Input: part model. Units: mm. Frame: model coordinates. Face numbers are marked on the shaded views. A direction names the side the tool comes from. Round coordinates to 2 decimals unless told otherwise and drop trailing zeros. Use a Markdown table: item, result.
Autodesk Fusion 360 part; units mm, degrees
sketch "Sketch1" plane through (0, 0, 0) normal (0, 0, 1) x (1, 0, 0)
  line L0 (50, 30) -> (20, 30)
  line L1 (0, 0) -> (20, 30)
  line L2 (50, 30) -> (70, 0)
  line L3 (0, 0) -> (10, -10)
  line L4 (10, -10) -> (60, -10)
  line L5 (60, -10) -> (70, 0)
ref_plane "WorkPlane1" through (0, 0, 100) normal (0, 0, 1) x (1, 0, 0)
sketch "Sketch2" plane through (0, 0, 100) normal (0, 0, 1) x (1, 0, 0)
  line L0 (30, 10) -> (40, 10)
  line L1 (60, -20) -> (10, -20)
  line L2 (30, 10) -> (5, -15)
  line L3 (5, -15) -> (10, -20)
  line L4 (40, 10) -> (65, -15)
  line L5 (65, -15) -> (60, -20)
loft "Loft1" add profiles "Sketch1", "Sketch2" section 1 section 2 makes body 1
ref_plane "WorkPlane2" through (35, 10, 50) normal (0, 0, -1) x (-1, 0, 0)
sketch "Sketch3" plane through (0, 0, 50) normal (0, 0, -1) x (-1, 0, 0)
  line L0 (0.4452, 9.35) -> (-20, 9.35)
  line L1 (-20, 9.35) -> (-20, -30.9261)
  line L2 (-20, -30.9261) -> (0.4452, -30.9261)
  line L3 (0.4452, -30.9261) -> (0.4452, 9.35)
  line L4 (-69.0117, 9.35) -> (-50, 9.35)
  line L5 (-50, 9.35) -> (-50, -30.2583)
  line L6 (-50, -30.2583) -> (-69.0117, -30.2583)
  line L7 (-69.0117, -30.2583) -> (-69.0117, 9.35)
extrude "Extrude1" cut sketch "Sketch3" along normal blind -6 and the other way blind -6 bodies 1
ref_plane "WorkPlane3" through (35, 10, -15.5) normal (0, 0, -1) x (-1, 0, 0)
sketch "Sketch4" plane through (0, 0, -15.5) normal (0, 0, -1) x (-1, 0, 0)
  line L0 (-70, 0) -> (-60, 15)
  line L1 (0, 0) -> (-10, -10)
  line L2 (-10, -10) -> (-60, -10)
  line L3 (-60, -10) -> (-70, 0)
  line L4 (-10, 15) -> (0, 0)
  line L5 (-60, 15) -> (-10, 15)
extrude "Extrude2" add sketch "Sketch4" along normal blind 5 separate body makes body 2
sketch "Sketch5" plane through (0, 0, 0) normal (0, 0, -1) x (1, 0, 0)
  line L0 (10, 10) -> (0, 0)
  line L1 (0, 0) -> (20, -30)
  line L2 (20, -30) -> (50, -30)
  line L3 (50, -30) -> (70, 0)
  line L4 (70, 0) -> (60, 10)
  line L5 (60, 10) -> (10, 10)
  line L6 (10, 10) -> (60, 10)
  line L7 (60, 10) -> (60, 0)
  line L8 (60, 0) -> (10, 0)
  line L9 (10, 0) -> (10, 10)
extrude "Extrude3" add sketch "Sketch5" along normal blind 20 contours L5 L6 L7 L8 L9 bodies 1 2
sketch "Sketch6" plane through (0, 0, 100) normal (0, 0, 1) x (-1, 0, 0)
  line L0 (-5, 15) -> (-10, 20)
  line L1 (-10, 20) -> (-60, 20)
  line L2 (-60, 20) -> (-65, 15)
  line L3 (-65, 15) -> (-40, -10)
  line L4 (-40, -10) -> (-30, -10)
  line L5 (-30, -10) -> (-5, 15)
  line L6 (-20, 0) -> (-50, 0)
  line L7 (-50, 0) -> (-50, 20)
  line L8 (-50, 20) -> (-20, 20)
  line L9 (-20, 20) -> (-20, 0)
extrude "Extrude4" add sketch "Sketch6" along normal blind 20 contours L1 L6 L7 L8 L9 bodies 1
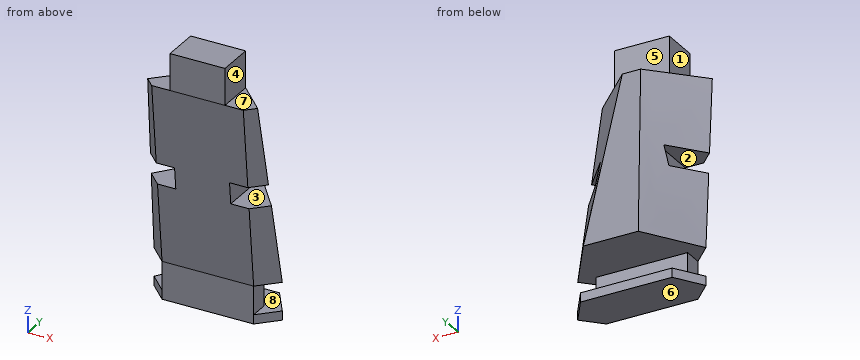
1) Draft query along Z for the marked faces 5, 6, 7 and 8. Return one class per face: released by +Z, released by -Z, zero draft, split by the parting line, or undercut.
Answer key:
| item | result |
|---|---|
| face 5 | zero draft |
| face 6 | released by -Z |
| face 7 | released by +Z |
| face 8 | undercut |
2) Ray query, probe 1 along Z at (x, y) = (24.5, 1.5); probe 2 along Z at (x, y) = (51, -6.5); probe 3 along X at (y, z) = (-1, -8). Return the intervals inside material, ascending.
Answer key:
| item | result |
|---|---|
| probe 1 | z = -20.5 to -15.5, 0 to 100 |
| probe 2 | z = -20.5 to 44, 56 to 100 |
| probe 3 | x = 10 to 60 |
3) Set-up query: the marked faces 1, 2, 3 and 4. Return all of +Z, -Z, +X, -X, +Y, -Y with unobstructed straight access to the full face (end or side cutting, diameter ignored); none if empty.
Answer key:
| item | result |
|---|---|
| face 1 | +Z, -X, +Y, -Y |
| face 2 | -X, -Y |
| face 3 | +X, -Y |
| face 4 | +Z, +X, +Y, -Y |
4) Cut plane A-A on x = 63. State how many separate pieces and enclosed holes the cut face has, and give its area (3 significant figures).
Answer key:
| item | result |
|---|---|
| separate pieces | 3 |
| enclosed holes | 0 |
| area | 992 mm^2 |
5) Contact query for flat-ended pins moving along their axis: P1, Ø5.5, axis at x = 51.5, z = 50, coming from the -Y side; P2, Ø5, axis at y = 3.5, z = 14.5, coming from the -X side; P3, Ø2, axis at x = 7.5, z = 79.5, coming from the -Y side (3 decimals). Output: stop coordinate, or through.
Answer key:
| item | result |
|---|---|
| P1 | stops at y = -15.23 |
| P2 | stops at x = 2.93 |
| P3 | stops at y = -16.455 |
